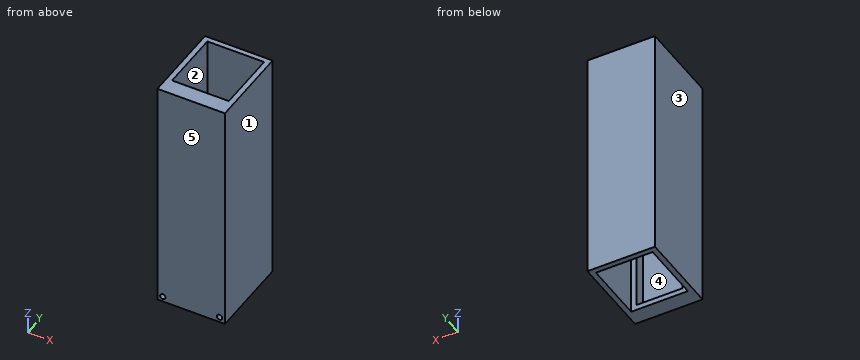
from build123d import *

# Parameters (mm, degrees)
SKETCH1_W           = 53.975
SKETCH1_H           = 165.1
SKETCH1_H_2         = 93.6625
BOSS_EXTRUDE4_DEPTH = 12.7
SKETCH4_W           = 66.675
SKETCH4_H           = 6.35
BOSS_EXTRUDE5_DEPTH = 277.8125
BOSS_EXTRUDE6_DEPTH = 277.8125
SKETCH6_R           = 3.175
CUT_EXTRUDE3_DEPTH  = 6.35


with BuildPart() as part:
    # Sketch1 → Boss-Extrude4 (new body)
    with BuildSketch(Plane(origin=(0, 0, 0), x_dir=(1, 0, 0), z_dir=(0, 1, 0))):
        Polygon((33.3375, -88.9), (33.3375, 88.9), (33.3375, 188.9125), (-33.3375, 188.9125), (-33.3375, 88.9), (-33.3375, -88.9), align=None)
        Rectangle(SKETCH1_W, SKETCH1_H, mode=Mode.SUBTRACT)
        with Locations((0, 135.73125)):
            Rectangle(SKETCH1_W, SKETCH1_H_2, mode=Mode.SUBTRACT)
    extrude(amount=BOSS_EXTRUDE4_DEPTH)

    # Sketch4 → Boss-Extrude5 (add)
    with BuildSketch(Plane.XY.offset(88.9)):
        with Locations((0, -3.175)):
            Rectangle(SKETCH4_W, SKETCH4_H)
    extrude(amount=-BOSS_EXTRUDE5_DEPTH)

    # Sketch5 → Boss-Extrude6 (add)
    with BuildSketch(Plane.XY.offset(88.9)):
        Polygon((-39.6875, -6.35), (-39.6875, 91.44), (39.6875, 91.44), (39.6875, -6.35), (33.3375, -6.35), (33.3375, 85.09), (-33.3375, 85.09), (-33.3375, -6.35), align=None)
    extrude(amount=-BOSS_EXTRUDE6_DEPTH)

    # Sketch6 → Cut-Extrude3 (cut)
    with BuildSketch(Plane.XZ.offset(6.35)):
        with Locations(Location((-33.3375, -182.5625, 0), (0, 0, 270))):
            Circle(SKETCH6_R)
        with Locations(Location((33.3375, -182.5625, 0), (0, 0, 90))):
            Circle(SKETCH6_R)
    extrude(amount=-CUT_EXTRUDE3_DEPTH, mode=Mode.SUBTRACT)


solid = part.part
Check sheet for the modelled part. Datum: model origin and axes. Units: mm. Face numbers are marked on the shaded views. A direction names the side the tool comes from. Round coordinates to 2 decimals unless told otherwise and drop trailing zeros. Order: outer loops, then holes, each group sorted by start corner. A loop starts at its lowest first (then second) coordinate and runs counter-clockwise, first axis right, second up. Notation, with made-up numbers: M 79.25,42.5 L 95.25,42.5 A17 cw 95.25,67.5 Z; hole C -29,-35.5 d6. An arc over 180 degrees is marked long. One line per item, written item: value. Start each with the question number.
1. Section check B-B on x = 3. Enter the section's corners in (y, z).
2. Scan lines: line 1 along Z through (x, y) = (-12, 3); line 2 along X through (y, z) = (2, -26); line 3 along Y through (x, z) = (23.5, 53). Record each from-to range of solid material in increasing order.
3. Section check C-C on z = 4. Enter the section's corners in (x, y), and give its area (3 significant figures).
4. Section check A-A on y = 22. Enter the section's corners in (x, z), and give its area (3 significant figures).
5. Access from +Z, -Z, +X, -X, +Y, -Y to the whole of each face (thin tool, end or side, straight path). Record for the marked faces 1 and 2.
6. Release check for a two-part mould opening along Y. For the marked faces 3, 4 and 5 record: released by +Y, released by -Y, zero draft, split by the parting line, or undercut.
Results found:
1. outline: M -6.35,-188.91 L 12.7,-188.91 L 12.7,-182.56 L 0,-182.56 L 0,-88.9 L 12.7,-88.9 L 12.7,-82.55 L 0,-82.55 L 0,82.55 L 12.7,82.55 L 12.7,88.9 L -6.35,88.9 Z; M 85.09,-188.91 L 91.44,-188.91 L 91.44,88.9 L 85.09,88.9 Z
2. line 1: -188.91 to -182.56, -88.9 to -82.55, 82.55 to 88.9
2. line 2: -39.69 to -26.99, 26.99 to 39.69
2. line 3: -6.35 to 0, 85.09 to 91.44
3. outline: M -39.69,-6.35 L 39.69,-6.35 L 39.69,91.44 L -39.69,91.44 Z; hole M -33.34,12.7 L -26.99,12.7 L -26.99,0 L 26.99,0 L 26.99,12.7 L 33.34,12.7 L 33.34,85.09 L -33.34,85.09 Z
3. area: 2,250 mm^2
4. outline: M -39.69,-188.91 L -33.34,-188.91 L -33.34,88.9 L -39.69,88.9 Z; M 33.34,-188.91 L 39.69,-188.91 L 39.69,88.9 L 33.34,88.9 Z
4. area: 3,530 mm^2
5. face 1: +Z, -Z, +X, +Y, -Y
5. face 2: +Z, -Z
6. face 3: zero draft
6. face 4: undercut
6. face 5: released by -Y
